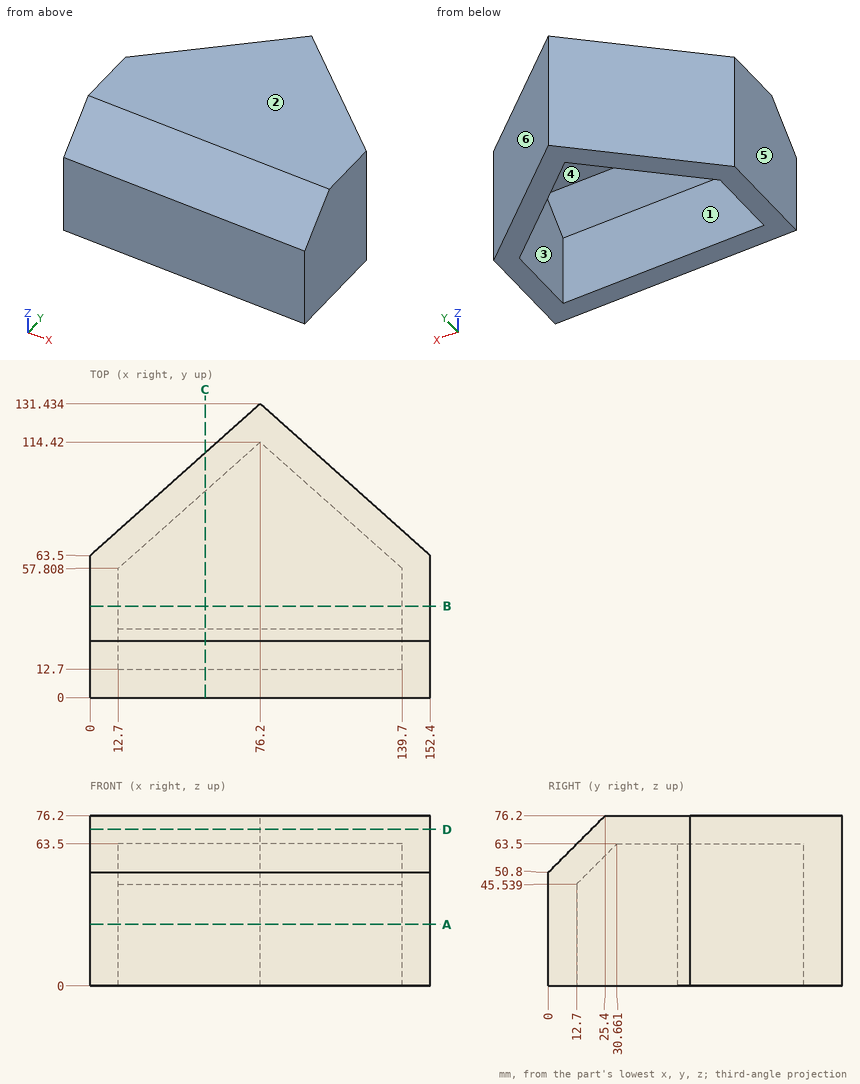
Can you work these out from the drawing? Everything is in mm from the part's minimum corner. A direction names the side the tool comes from. Coordinates: 2 decimals unless noted, no trailing zeros. Loops run counter-clockwise (first coordinate to the right, second up) from the corner with the lowest first, then second, coordinate; pieces in that order, holes last. Notation, with made-up numbers: M 50,-20 L 85,-20 A33 cw 85,11 Z; hole C 55,52 d8. An arc over 180 degrees is marked long. Put each result on its own line as item: value. Start each with the question number.
(1) Suppose I cut it at D-D on z = 70. Please give me the cut outline in (x, y), then the cut area to 3 significant figures.
(2) Suppose I cut it at C-C on x = 51.5. Please give me the cut outline in (y, z).
(3) Suppose I cut it at B-B on y = 41. Please give me the cut outline in (x, z).
(4) Will these pins go through, and if not, where does the flat tip stop? P1, Ø3, axis at x = 37, y = 60, coming from the -Z side; P2, Ø2, axis at x = 29.5, z = 33, coming from the +Y side; P3, Ø3, axis at x = 78.5, z = 59, coming from the +Y side; P4, Ø1.5, axis at x = 115.5, y = 99, coming from the +Z side.
(5) Suppose I cut it at A-A on z = 27.5. Please give me the cut outline in (x, y).
(6) Thinking about a two-plate mould opening in Y: for the marked faces 3, 4, 5 and 6, which applies, pulls with the +Y half, pulls with the -Y half, needs draft (parallel to the pull), parting line crosses it, or undercut?
(7) For the marked faces 1 and 2, which set-ups out of +Z, -Z, +X, -X, +Y, -Y let a thin tool reach every point of the face, with its end or its side?
(8) I need wall thicknesses on line 1 (X direction, y = 50.5, z = 57.5); line 2 (Z direction, x = 13, y = 37.5); line 3 (Y direction, x = 48, z = 16) (1 decimal). Which ranges of each line are inside material? Lowest first, please. Write a range as from..to.
Solutions:
1. outline: M 0,19.2 L 152.4,19.2 L 152.4,63.5 L 76.2,131.43 L 0,63.5 Z
1. area: 11,900 mm2
2. outline: M 0,0 L 12.7,0 L 12.7,45.54 L 30.66,63.5 L 92.4,63.5 L 92.4,0 L 109.41,0 L 109.41,76.2 L 25.4,76.2 L 0,50.8 Z
3. outline: M 0,0 L 12.7,0 L 12.7,63.5 L 139.7,63.5 L 139.7,0 L 152.4,0 L 152.4,76.2 L 0,76.2 Z
4. P1: stops at z = 63.5
4. P2: stops at y = 90.69
4. P3: stops at y = 130.72
4. P4: passes through
5. outline: M 0,0 L 152.4,0 L 152.4,63.5 L 76.2,131.43 L 0,63.5 Z; hole M 12.7,12.7 L 139.7,12.7 L 139.7,57.81 L 76.2,114.42 L 12.7,57.81 Z
6. face 3: undercut
6. face 4: undercut
6. face 5: needs draft
6. face 6: pulls with the +Y half
7. face 1: -Z
7. face 2: +Z, +X, -X, +Y, -Y
8. line 1: x = 0..12.7, 139.7..152.4
8. line 2: z = 63.5..76.2
8. line 3: y = 0..12.7, 89.3..106.3
